Here's how the part is built. I have some questions about the finished solid (model axes, mm). Face numbers are marked on the shaded views. Give positions to 0.01 mm unless a question says otherwise; leave off trailing zeros. Write each loop counter-clockwise with the first axis right and the second up, starting at its lowest first coordinate (ties: lowest second). Pieces come first, ordered by that corner, then holes. Notation, with made-up numbers: (35, -36.75) - (52, -36.75) arc R26 ccw to (52, -15.75) - close; hole circle Ø8 at (-17, 68). An arc over 180 degrees is marked (long way). One line per item, written item: value. Start each with the question number.
1) Please list where these lines run through material, in increasing order: L1, parallel to Y at x = 0, z = 7; L2, parallel to Y at x = 2.25, z = 7.25; L3, parallel to X at y = -5.25, z = 7.15. Write a range as [from, to].
2) Imagine slicing it at C-C on z = 6.55. Write out the boundary of the cut face in (x, y), plus the area to 3 significant figures.
3) We'd pull the mould along X, two halves only. Please class the marked faces 1 and 2: +X half, -X half, draft (parallel to the pull), parting line (faces both ways), or undercut.
4) Imagine slicing it at A-A on y = 0. Write out the boundary of the cut face in (x, z), plus the area to 3 significant figures.
5) I'm going to push a flat-ended pin straight in: P1, Ø4.5, axis at x = 0, y = 0, coming from the -Z side. Where does the tip first touch, or does it pass through?
from build123d import *

# Parameters (mm, degrees)
SKETCH001_R  = 7.75
PAD_DEPTH    = 1
FILLET_R     = 0.5
SKETCH002_R  = 2.5
POCKET_DEPTH = 5


with BuildPart() as part:
    # Sketch001 (on Face1 of CopyInvoluteGear) → Pad (new body)
    with BuildSketch(Plane.XY.offset(6.3)):
        Circle(SKETCH001_R)
    extrude(amount=PAD_DEPTH)

    # Fillet
    fillet_edges = [part.edges().sort_by_distance(p)[0] for p in [
        (-7.75, 0, 6.3),
    ]]
    fillet(fillet_edges, radius=FILLET_R)

    # Sketch002 (on Face3 of Fillet) → Pocket (cut)
    with BuildSketch(Plane.XY.offset(7.3)):
        Circle(SKETCH002_R)
    extrude(amount=-POCKET_DEPTH, mode=Mode.SUBTRACT)


solid = part.part
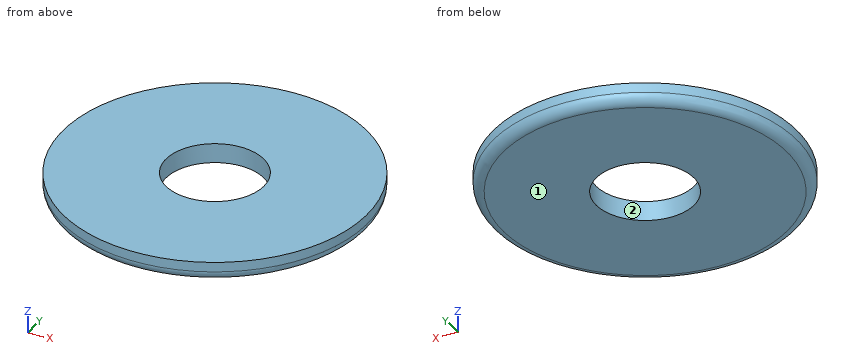
Numbers:
1. L1: [-7.75, -2.5], [2.5, 7.75]
1. L2: [-7.42, -1.09], [1.09, 7.42]
1. L3: [-5.7, 5.7]
2. outline: circle Ø15.37 at (0, 0); hole circle Ø5 at (0, 0)
2. area: 166 mm^2
3. face 1: draft
3. face 2: undercut
4. outline: (-7.75, 6.8) arc R0.5 ccw to (-7.25, 6.3) - (-2.5, 6.3) - (-2.5, 7.3) - (-7.75, 7.3) - close; (2.5, 6.3) - (7.25, 6.3) arc R0.5 ccw to (7.75, 6.8) - (7.75, 7.3) - (2.5, 7.3) - close
4. area: 10.4 mm^2
5. P1: through
